Geometry check sheet. Reference: the model listing, model coordinates, mm. Round coordinates to 2 decimals unless told otherwise and drop trailing zeros. Loops run counter-clockwise (first coordinate to the right, second up) from the corner with the lowest first, then second, coordinate; pieces in that order, holes last. Notation, with made-up numbers: M -13.75,52.5 L 6.25,52.5 A21 cw 6.25,65.5 Z; hole C 35.25,-37.5 d10. An arc over 180 degrees is marked long. Use one line per item in the form item = value. Start each with the question number.
1. Draft check along Z on faces 1 (the flat face through (81, 7, -79)), 2 (the flat face through (102, 37, -104)), 3 (the flat face through (126, 7, -124)), 4 (the flat face through (102, 13, 0)). Enter one of: pulls with the +Z half, pulls with the -Z half, needs draft (parallel to the pull), parting line crosses it, or undercut.
2. Cross-section at B-B (x = 125.5). Record the boundary of the cut face in (y, z).
3. Material ranges on line 1 (Z direction, x = 35, y = 17); line 2 (X direction, y = 16, z = -163.5); line 3 (Z direction, x = 122, y = 19.5), recorded low to high.
4. Cross-section at A-A (y = 33.5). State how many separate pieces and enclosed holes the cut face has, then the cut area to 3 significant figures.
5. Cross-section at C-C (z = -36). Record the boundary of the cut face in (x, y), then the cut area to 3 significant figures.
6. Go/stop test with flat-tipped pins: pin 1 (12.5 mm diameter, centred on x = 165, z = -36, fed in from +Y); pin 2 (2 mm diameter, centred on x = 65.5, y = 30.5, fed in from -Z). Record where each tip stops, or that it passes through.
```python
from build123d import *

# Parameters (mm, degrees)
SKETCH1_W           = 206
SKETCH1_H           = 206
BOSS_EXTRUDE1_DEPTH = 37
SKETCH2_R           = 12.5
CUT_EXTRUDE1_DEPTH  = 30
LPATTERN1_COUNT     = 4
LPATTERN1_PITCH     = 45
FILLET2_R           = 10


with BuildPart() as part:
    # Sketch1 → Boss-Extrude1 (new body)
    with BuildSketch(Plane(origin=(0, 0, 0), x_dir=(1, 0, 0), z_dir=(0, 1, 0))):
        with Locations((103, 103)):
            Rectangle(SKETCH1_W, SKETCH1_H)
    extrude(amount=BOSS_EXTRUDE1_DEPTH)

    # Sketch2 → Cut-Extrude1 (cut)
    with BuildSketch(Plane(origin=(0, 37, 0), x_dir=(1, 0, 0), z_dir=(0, 1, 0))):
        with Locations(Location((80.5, 168.965188792, 0), (0, 0, 270))):
            Circle(SKETCH2_R)
        with Locations(Location((35.5, 168.965188792, 0), (0, 0, 270))):
            Circle(SKETCH2_R)
        with Locations(Location((125.5, 168.965188792, 0), (0, 0, 270))):
            Circle(SKETCH2_R)
        with Locations(Location((170.5, 168.965188792, 0), (0, 0, 270))):
            Circle(SKETCH2_R)
    cut_extrude1 = extrude(amount=-CUT_EXTRUDE1_DEPTH, mode=Mode.SUBTRACT)

    # LPattern1: Cut-Extrude1 ×4
    with Locations(*[(0, 0, i * LPATTERN1_PITCH) for i in range(1, LPATTERN1_COUNT)]):
        add(cut_extrude1, mode=Mode.SUBTRACT)

    # Fillet2
    fillet2_edges = [part.edges().sort_by_distance(p)[0] for p in [
        (206, 37, -103),
        (103, 37, -206),
        (0, 37, -103),
        (103, 37, 0),
    ]]
    fillet(fillet2_edges, radius=FILLET2_R)


solid = part.part
```
Reported:
q1.face_1 = undercut
q1.face_2 = needs draft
q1.face_3 = undercut
q1.face_4 = pulls with the +Z half
q2.outline = M 0,-206 L 27,-206 A10 ccw 37,-196 L 37,-181.47 L 7,-181.47 L 7,-156.47 L 37,-156.47 L 37,-136.47 L 7,-136.47 L 7,-111.47 L 37,-111.47 L 37,-91.47 L 7,-91.47 L 7,-66.47 L 37,-66.47 L 37,-46.47 L 7,-46.47 L 7,-21.47 L 37,-21.47 L 37,-10 A10 ccw 27,0 L 0,0 Z
q3.line_1 = -206 to -181.46, -156.48 to -136.46, -111.48 to -91.46, -66.48 to -46.46, -21.48 to 0
q3.line_2 = 0 to 24.26, 46.74 to 69.26, 91.74 to 114.26, 136.74 to 159.26, 181.74 to 206
q3.line_3 = -206 to -180.97, -156.97 to -135.97, -111.97 to -90.97, -66.97 to -45.97, -21.97 to 0
q4.separate_pieces = 1
q4.enclosed_holes = 16
q4.area = 32,600 mm²
q5.outline = M 0,0 L 206,0 L 206,27 A10 ccw 196,37 L 182.83,37 L 182.83,7 L 158.17,7 L 158.17,37 L 137.83,37 L 137.83,7 L 113.17,7 L 113.17,37 L 92.83,37 L 92.83,7 L 68.17,7 L 68.17,37 L 47.83,37 L 47.83,7 L 23.17,7 L 23.17,37 L 10,37 A10 ccw 0,27 Z
q5.area = 4,620 mm²
q6.pin_1 = 7
q6.pin_2 = -205.68
